Geometry: final body of the model. Coordinates: model frame, mm. A direction names the side the tool comes from. Coordinates: 2 decimals unless noted, no trailing zeros. Write each loop counter-clockwise with the first axis right and the second up, starting at its lowest first coordinate (ties: lowest second). Pieces come first, ordered by that corner, then holes. Notation, with made-up numbers: (80, -15.75) - (90, -15.75) arc R17 ccw to (90, 4.25) - close; hole circle Ø11 at (-3, 15). An arc over 180 degrees is marked (long way). Put each result on its own line as item: value.
```python
from build123d import *

# Parameters (mm, degrees)
BOSS_EXTRUDE1_DEPTH  = 2
FILLET1_R            = 3
CUT_EXTRUDE1_REACH   = 57.937
SKETCH2_R            = 1.25
SKETCH2_W            = 3
SKETCH2_H            = 22
FILLET2_R            = 1
FILLET2_OF_MIRROR1_R = 1
MIRROR2_OUTLINE_R    = 1.25
MIRROR2_DEPTH        = 2


# Read off the part's stored shape, not the designer's step: Mirror2
with BuildPart() as part:
    # Sketch1 → Boss-Extrude1 (new body)
    with BuildSketch(Plane(origin=(0, 0, 0), x_dir=(1, 0, 0), z_dir=(0, 1, 0))):
        Polygon((20, 50), (-20, 50), (-20, 40), (-25, 32.5), (-25, -32.5), (-20, -40), (-20, -50), (20, -50), (20, -40), (25, -32.5), (25, 32.5), (20, 40), align=None)
    extrude(amount=BOSS_EXTRUDE1_DEPTH)

    # Fillet1
    fillet1_edges = [part.edges().sort_by_distance(p)[0] for p in [
        (-20, 1, -50),
        (20, 1, -50),
        (20, 1, -40),
        (25, 1, -32.5),
        (25, 1, 32.5),
        (20, 1, 40),
        (20, 1, 50),
        (-20, 1, 50),
        (-20, 1, 40),
        (-25, 1, 32.5),
        (-25, 1, -32.5),
        (-20, 1, -40),
    ]]
    fillet(fillet1_edges, radius=FILLET1_R)

    # Sketch2 → Cut-Extrude1 (cut, up to next)
    with BuildSketch(Plane(origin=(0, 2, 0), x_dir=(1, 0, 0), z_dir=(0, 1, 0)), mode=Mode.PRIVATE) as cut_extrude1_sk1:
        with Locations(Location((12, 40, 0), (0, 0, 270))):
            Circle(SKETCH2_R)
    cut_extrude1_tool1 = extrude(cut_extrude1_sk1.sketch, amount=-CUT_EXTRUDE1_REACH, mode=Mode.PRIVATE) & part.part
    # Sketch2 → Cut-Extrude1 (cut, up to next)
    with BuildSketch(Plane(origin=(0, 2, 0), x_dir=(1, 0, 0), z_dir=(0, 1, 0)), mode=Mode.PRIVATE) as cut_extrude1_sk2:
        with Locations((21.5, 20)):
            Rectangle(SKETCH2_W, SKETCH2_H)
    cut_extrude1_tool2 = extrude(cut_extrude1_sk2.sketch, amount=-CUT_EXTRUDE1_REACH, mode=Mode.PRIVATE) & part.part
    # Sketch2 → Cut-Extrude1 (cut, up to next)
    with BuildSketch(Plane(origin=(0, 2, 0), x_dir=(1, 0, 0), z_dir=(0, 1, 0)), mode=Mode.PRIVATE) as cut_extrude1_sk3:
        with Locations((13.5, 18.5)):
            Rectangle(SKETCH2_W, SKETCH2_H)
    cut_extrude1_tool3 = extrude(cut_extrude1_sk3.sketch, amount=-CUT_EXTRUDE1_REACH, mode=Mode.PRIVATE) & part.part
    cut_extrude1_1 = cut_extrude1_tool1.solids().sort_by_distance((12, 2, -40))[0]
    add(cut_extrude1_1, mode=Mode.SUBTRACT)
    cut_extrude1_2 = cut_extrude1_tool2.solids().sort_by_distance((21.5, 2, -20))[0]
    add(cut_extrude1_2, mode=Mode.SUBTRACT)
    cut_extrude1_3 = cut_extrude1_tool3.solids().sort_by_distance((13.5, 2, -18.5))[0]
    add(cut_extrude1_3, mode=Mode.SUBTRACT)
    cut_extrude1 = cut_extrude1_1 + cut_extrude1_2 + cut_extrude1_3  # Cut-Extrude1 as one shape, for the pattern or mirror that repeats it

    # Fillet2
    fillet2_edges = [part.edges().sort_by_distance(p)[0] for p in [
        (20, 1, -9),
        (20, 1, -31),
        (23, 1, -31),
        (23, 1, -9),
        (15, 1, -29.5),
        (15, 1, -7.5),
        (12, 1, -7.5),
        (12, 1, -29.5),
    ]]
    fillet(fillet2_edges, radius=FILLET2_R)

    # Mirror1: Cut-Extrude1 across plane
    add(cut_extrude1.mirror(Plane.XY), mode=Mode.SUBTRACT)

    # Fillet2 of Mirror1
    fillet2_of_mirror1_edges = [part.edges().sort_by_distance(p)[0] for p in [
        (20, 1, 9),
        (20, 1, 31),
        (23, 1, 31),
        (23, 1, 9),
        (15, 1, 29.5),
        (15, 1, 7.5),
        (12, 1, 7.5),
        (12, 1, 29.5),
    ]]
    fillet(fillet2_of_mirror1_edges, radius=FILLET2_OF_MIRROR1_R)

    # Mirror2 outline → Mirror2 (cut)
    with BuildSketch(Plane(origin=(0, 0, 0), x_dir=(1, 0, 0), z_dir=(0, 1, 0))):
        with BuildLine():
            Line((-20, 10), (-20, 30))
            ThreePointArc((-20, 30), (-20.292893219, 30.707106781), (-21, 31))
            Line((-21, 31), (-22, 31))
            ThreePointArc((-22, 31), (-22.707106781, 30.707106781), (-23, 30))
            Line((-23, 30), (-23, 10))
            ThreePointArc((-23, 10), (-22.707106781, 9.292893219), (-22, 9))
            Line((-22, 9), (-21, 9))
            ThreePointArc((-21, 9), (-20.292893219, 9.292893219), (-20, 10))
        make_face()
        with BuildLine():
            ThreePointArc((-21, -31), (-20.292893219, -30.707106781), (-20, -30))
            Line((-20, -30), (-20, -10))
            ThreePointArc((-20, -10), (-20.292893219, -9.292893219), (-21, -9))
            Line((-21, -9), (-22, -9))
            ThreePointArc((-22, -9), (-22.707106781, -9.292893219), (-23, -10))
            Line((-23, -10), (-23, -30))
            ThreePointArc((-23, -30), (-22.707106781, -30.707106781), (-22, -31))
            Line((-22, -31), (-21, -31))
        make_face()
        with BuildLine():
            Line((-14, 7.5), (-13, 7.5))
            ThreePointArc((-13, 7.5), (-12.292893219, 7.792893219), (-12, 8.5))
            Line((-12, 8.5), (-12, 28.5))
            ThreePointArc((-12, 28.5), (-12.292893219, 29.207106781), (-13, 29.5))
            Line((-13, 29.5), (-14, 29.5))
            ThreePointArc((-14, 29.5), (-14.707106781, 29.207106781), (-15, 28.5))
            Line((-15, 28.5), (-15, 8.5))
            ThreePointArc((-15, 8.5), (-14.707106781, 7.792893219), (-14, 7.5))
        make_face()
        with BuildLine():
            ThreePointArc((-15, -28.5), (-14.707106781, -29.207106781), (-14, -29.5))
            Line((-14, -29.5), (-13, -29.5))
            ThreePointArc((-13, -29.5), (-12.292893219, -29.207106781), (-12, -28.5))
            Line((-12, -28.5), (-12, -8.5))
            ThreePointArc((-12, -8.5), (-12.292893219, -7.792893219), (-13, -7.5))
            Line((-13, -7.5), (-14, -7.5))
            ThreePointArc((-14, -7.5), (-14.707106781, -7.792893219), (-15, -8.5))
            Line((-15, -8.5), (-15, -28.5))
        make_face()
        with Locations((-12, 40)):
            Circle(MIRROR2_OUTLINE_R)
        with Locations((-12, -40)):
            Circle(MIRROR2_OUTLINE_R)
    extrude(amount=MIRROR2_DEPTH, mode=Mode.SUBTRACT)


solid = part.part
```
1. Pin query (flat end, axial travel): pin 1 Ø1.1 at (x, y) = (-21.5, 1) entering from -Z (3 decimals); pin 2 Ø1.5 at (x, z) = (12, 40) entering from -Y; pin 3 Ø1.1 at (x, y) = (-21.5, 1) entering from +Z (3 decimals); pin 4 Ø1.5 at (x, z) = (-16.5, -26.5) entering from -Y. Return the tip coordinate at first contact, or that it passes through.
Answer below:
pin 1: stops at z = -38.575
pin 2: passes through
pin 3: stops at z = 38.575
pin 4: stops at y = 0
2. Set-up query: faces 4 (the flat face through (-20, 1, -44)), 5 (the flat face through (0, 2, -1)), 6 (the flat face through (-23, 1, 20)). Return all of +Z, -Z, +X, -X, +Y, -Y with unobstructed straight access to the full face (end or side cutting, diameter ignored); none if empty.
Answer below:
face 4: -Z, -X, +Y, -Y
face 5: +Z, -Z, +X, -X, +Y
face 6: +Y, -Y
3. Mould query, pull axis X, two halves, no side actions, for faces 1 (the flat face through (0, 1, 50)), 2 (the cylindrical face through (-13.25, 0.99, 39.95)), 3 (the flat face through (20, 1, 44)). Classes: +X half, -X half, draft (parallel to the pull), parting line (faces both ways), or undercut.
Answer below:
face 1: draft
face 2: undercut
face 3: +X half
4. Ray query, probe 1 along X at (y, z) = (0.1, -19.5); probe 2 along X at (y, z) = (0.9, -40); probe 3 along X at (y, z) = (1.4, -45). Return the intervals inside material, ascending. Write a range as from..to.
Answer below:
probe 1: x = -25..-23, -20..-15, -12..12, 15..20, 23..25
probe 2: x = -20.14..-13.25, -10.75..10.75, 13.25..20.14
probe 3: x = -20..20
5. Section query A-A (z = -21). Return loops of the section in (x, y), then the cut area to 3 significant figures.
Answer below:
outline: (-25, 0) - (-23, 0) - (-23, 2) - (-25, 2) - close; (-20, 0) - (-15, 0) - (-15, 2) - (-20, 2) - close; (-12, 0) - (12, 0) - (12, 2) - (-12, 2) - close; (15, 0) - (20, 0) - (20, 2) - (15, 2) - close; (23, 0) - (25, 0) - (25, 2) - (23, 2) - close
area: 76.0 mm²
6. Section query B-B (y = 0.7). Count the separate pieces of the cut face and the enclosed holes in it, then the cut area to 3 significant figures.
Answer below:
separate pieces: 1
enclosed holes: 12
area: 4,180 mm²
